Build history of the part. All positions in model axes, mm. Round coordinates to 2 decimals unless told otherwise and drop trailing zeros. Order: outer loops, then holes, each group sorted by start corner. A loop starts at its lowest first (then second) coordinate and runs counter-clockwise, first axis right, second up. Notation, with made-up numbers: M -24.5,-35.5 L 15.5,-35.5 A15 ccw 15.5,-26.5 Z; hole C -30.75,65 d11. An arc over 180 degrees is marked long. Use CSV: the item, a comma, the result in double quotes.
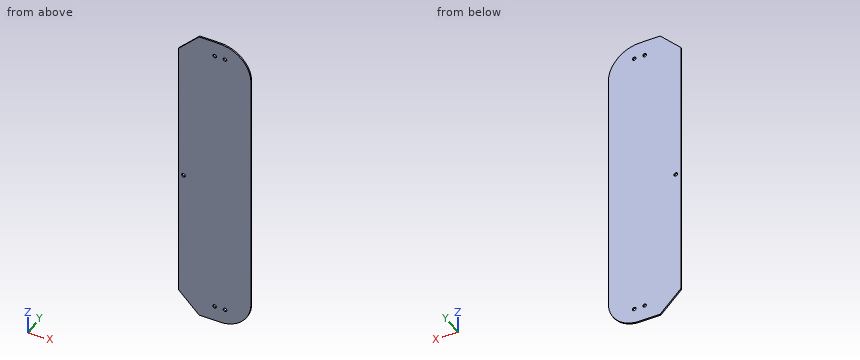
Autodesk Inventor part; units mm, degrees
ref_plane "YZ Plane" through (0, 0, 0) normal (1, 0, 0) x (0, 1, 0)
ref_plane "XZ Plane" through (0, 0, 0) normal (0, 1, 0) x (-1, 0, 0)
ref_plane "XY Plane" through (0, 0, 0) normal (0, 0, 1) x (1, 0, 0)
sketch "Sketch1" plane through (0, 0, 0) normal (0, 1, 0) x (-1, 0, 0)
  line L0 (0, 0) -> (-12.7, 0)
  line L1 (-50.8, 38.1) -> (-50.8, 342.9)
  line L2 (-12.7, 381) -> (0, 381)
  line L3 (0, 0) -> (12.7, 0)
  line L4 (38.1, 25.4) -> (38.1, 355.6)
  line L5 (12.7, 381) -> (0, 381)
  arc A0 (-12.7, 381) -> (-50.8, 342.9) centre (-12.7, 342.9) ccw
  arc A1 (-50.8, 38.1) -> (-12.7, 0) centre (-12.7, 38.1) ccw
  line L6 (38.1, 355.6) -> (12.7, 381)
  line L7 (38.1, 25.4) -> (12.7, 0)
  circle A2 centre (31.75, 184.15) radius 2.2225
  circle A3 centre (-6.35, 19.05) radius 2.2225
  circle A4 centre (-19.05, 19.05) radius 2.2225
  circle A5 centre (-6.35, 361.95) radius 2.2225
  circle A6 centre (-19.05, 361.95) radius 2.2225
  point P0 (-50.8, 381)
  point P1 (-50.8, 0)
  point P2 (38.1, 381)
  point P3 (38.1, 0)
  dimension "d0" = 50.8
  dimension "d1" = 381
  dimension "d2" = 38.1
  dimension "d3" = 381
  dimension "d4" = 38.1
  dimension "d5" = 25.4
  dimension "d6" = 25.4
  dimension "d7" = 25.4
  dimension "d8" = 25.4
  dimension "d12" = 4.445
  dimension "d13" = 4.445
  dimension "d14" = 4.445
  dimension "d15" = 4.445
  dimension "d16" = 4.445
extrude "Extrusion1" add sketch "Sketch1" along normal blind 1.778
properties part number "side_ring_guard"
(1) Drop a flat-ended pin along its axis: pin 1 (3.5 mm diameter, centred on x = -31.75, z = 184.15, fed in from +Y). Give the stop position or say it passes through.
Answer block:
pin 1,"passes through"
(2) Wall check: line 1 (Z direction, x = 6.35, y = 0.9); line 2 (Z direction, x = 19.05, y = 0.7); line 3 (X direction, y = 1, z = 184.15). Give the ranges that are in metal, low to high. Write a range as from..to.
Answer block:
line 1,"z = 0..16.83, 21.27..359.73, 364.17..381"
line 2,"z = 0.53..16.83, 21.27..359.73, 364.17..380.47"
line 3,"x = -38.1..-33.97, -29.53..50.8"
(3) Cut at A-A, the plane y = 0.7. Count the separate pieces of the cut face and the enclosed holes in it, and give its area (3 significant figures).
Answer block:
separate pieces,"1"
enclosed holes,"5"
area,"32,500 mm²"
(4) Cut at B-B, the plane x = 42. Give the cut face in (y, z), and give its area (3 significant figures).
Answer block:
outline,"M 0,13.75 L 1.78,13.75 L 1.78,367.25 L 0,367.25 Z"
area,"629 mm²"
